```python
from build123d import *

# Parameters (mm, degrees)
CROQUIS2_R              = 4.5
SALIENTE_EXTRUIR2_DEPTH = 10
CHAFL_N1_SIZE           = 5


with BuildPart() as part:
    # Croquis2 → Saliente-Extruir2 (new body)
    with BuildSketch(Plane(origin=(0, 0, 0), x_dir=(1, 0, 0), z_dir=(0, 1, 0))):
        with BuildLine():
            Line((-91.379241818, 5.129552955), (-91.379241818, 18.223049557))
            Line((-91.379241818, 18.223049557), (-122.718097219, 0.129552955))
            Line((-122.718097219, 0.129552955), (-91.379241818, -17.963943646))
            Line((-91.379241818, -17.963943646), (-91.379241818, -4.870447045))
            Line((-91.379241818, -4.870447045), (83.871392309, -4.870447045))
            ThreePointArc((83.871392309, -4.870447045), (123.23630904, 0.129552955), (83.871392309, 5.129552955))
            Line((83.871392309, 5.129552955), (-91.379241818, 5.129552955))
        make_face()
        with Locations(Location((103.23630904, 0.129552955, 0), (0, 0, 270))):
            Circle(CROQUIS2_R, mode=Mode.SUBTRACT)
    extrude(amount=SALIENTE_EXTRUIR2_DEPTH)

    # Chaflán1
    chafl_n1_edges = [part.edges().sort_by_distance(p)[0] for p in [
        (-107.048669518, 10, -9.176301256),
        (-107.048669518, 10, 8.917195345),
        (103.23630904, 10, -4.629552955),
        (-91.379241818, 10, 11.417195345),
        (-3.753924755, 10, 4.870447045),
        (123.23630904, 10, -0.129552955),
        (-3.753924755, 10, -5.129552955),
        (-91.379241818, 10, -11.676301256),
    ]]
    chamfer(chafl_n1_edges, length=CHAFL_N1_SIZE - 0.0001)  # a hair under: the kernel refuses the full size


solid = part.part
```
Geometry check sheet. Reference: the model listing, model coordinates, mm. A direction names the side the tool comes from. Round coordinates to 2 decimals unless told otherwise and drop trailing zeros. Loops run counter-clockwise (first coordinate to the right, second up) from the corner with the lowest first, then second, coordinate; pieces in that order, holes last. Notation, with made-up numbers: (16.25, 22) - (25.25, 22) arc R21 ccw to (25.25, 26) - close; hole circle Ø6 at (71, -35.5). An arc over 180 degrees is marked (long way). Write each question's results on one line, items separated by ' | '. Start each with the question number.
Q1. Gauge pin test, flat ends, axial feed: P1, Ø5.5, axis at y = 3.5, z = 14.5, coming from the +X side; P2, Ø5.5, axis at y = 1.5, z = -9, coming from the +X side; P3, Ø5.5, axis at x = -10, y = 3.5, coming from the +Z side; P4, Ø2, axis at y = 3, z = -1, coming from the -X side. Record the tip position at first contact, or that the pin passes through.
Q2. Release check for a two-part mould opening along Z. For faces 1 (the flat face through (-107.27, 2.47, 8.79)), 2 (the cylindrical face through (99.244, 2.465, 1.947)), 3 (the conical face through (108.008, 5.313, -0.756)), 4 (the conical face through (118.46, 9.76, 0.54)) record: +Z half, -Z half, draft (parallel to the pull), parting line (faces both ways), or undercut.
Q3. Cross-section at A-A on y = 7.25. Enter the section's corners in (x, z), and give its area (3 significant figures).
Q4. Access from +Z, -Z, +X, -X, +Y, -Y to the whole of each face (thin tool, end or side, straight path). Record for faces 5 (the flat face through (-91.379, 2, -12)), 6 (the flat face through (-93.914, 7.535, 9.044)), 7 (the flat face through (-5, 2, 4.87)).
Q5. Thickness scan on line 1 (X direction, y = 8.5, z = -3); line 2 (Z direction, x = 103, y = 1.5); line 3 (X direction, y = 8.25, z = -6.5). Record the ranges inside material, lowest first. Write a range as [from, to].
Answers below:
1) P1: stops at x = 119.33 | P2: stops at x = 122.28 | P3: stops at z = 4.87 | P4: stops at x = -122.72
2) face 1: +Z half | face 2: undercut | face 3: undercut | face 4: parting line
3) outline: (-118.22, -0.13) - (-93.63, -14.33) - (-93.63, -2.88) - (85.7, -2.88) arc R17.75 ccw (long way) to (85.7, 2.62) - (-93.63, 2.62) - (-93.63, 14.07) - close; hole circle Ø13.5 at (103.24, -0.13) | area: 2,180 mm²
4) face 5: -Z, +Y, -Y | face 6: +Z, +Y | face 7: +Z, +Y, -Y
5) line 1: x = [-110.75, -94.88], [86.99, 95.77], [110.7, 119.48] | line 2: z = [-20.13, -4.62], [4.36, 19.87] | line 3: x = [-105.18, -94.63], [87.74, 98.82], [107.65, 118.73]
